Here's how the part is built. I have some questions about the finished solid (model axes, mm). A direction names the side the tool comes from. Coordinates: 2 decimals unless noted, no trailing zeros. Write each loop counter-clockwise with the first axis right and the second up, starting at its lowest first coordinate (ties: lowest second). Pieces come first, ordered by that corner, then holes. Notation, with made-up numbers: M 68.5,-35 L 102.5,-35 A30 ccw 102.5,-6 Z; hole C -23.5,29 d8. An arc over 180 degrees is marked long. Use one line per item in the form item = value. Start each with the question number.
1. On a 3-axis mill with a long thin cutter (end or side, diameter ignored), from which of +Z, -Z, +X, -X, +Y, -Y can I reach the whole of each face in a straight line? I mean faces 1 (the face through (-3.84, -3.97, -6.54)), 2 (the face through (-54, -1, -10)), 3 (the face through (-107.134, -8.541, -8.468)), 4 (the face through (2.51, 2.24, -8.47)), 5 (the face through (-53, -1, -13)). Say none if no direction works.
2. I want a section at B-B, the plane x = -19.5. List the corners of the cut face in (y, z) for me, plus the area to 3 significant figures.
3. Please list where these lines run through material, in increasing order: line 1 along Z through (x, y) = (-76.5, -0.5); line 2 along X through (y, z) = (-0.25, -1) (3 decimals); line 3 along Y through (x, z) = (-60, -11.5). Write a range as [from, to].
4. I'm going to push flat-ended pins straight in: pin 1 Ø1.1 at (x, z) = (-5.5, -6.5) entering from -Y; pin 2 Ø1.4 at (x, y) = (-109.5, -8) entering from -Z; pin 3 Ø8 at (y, z) = (-5.5, -9.5) entering from +X. Where does each tip first touch, or does it pass through?
5. Thinking about a two-plate mould opening in Y: for faces 6 (the face through (-108.25, -4, -9)), 7 (the face through (-109, -4, -10.75)), 8 (the face through (-55, -2, -11)), which applies, released by +Y, released by -Y, zero draft, split by the parting line, or undercut?
6. I want a section at C-C, the plane y = -3.5. List the corners of the cut face in (x, z) for me, plus the area to 3 significant figures.
7. I want a section at A-A, the plane z = -2.25. List the corners of the cut face in (x, y) for me (3 decimals).
Autodesk Inventor part; units mm, degrees
ref_plane "YZ Plane" through (0, 0, 0) normal (1, 0, 0) x (0, 1, 0)
ref_plane "XZ Plane" through (0, 0, 0) normal (0, 1, 0) x (-1, 0, 0)
ref_plane "XY Plane" through (0, 0, 0) normal (0, 0, 1) x (1, 0, 0)
sketch "Skizze1" plane through (0, 0, 0) normal (0, 1, 0) x (-1, 0, 0)
  line L0 (0, 0) -> (108, 0)
  line L1 (108, 0) -> (108, -15)
  line L2 (108, -15) -> (0, -15)
  line L3 (0, -15) -> (0, 0)
  dimension "d0" = 108
  dimension "d1" = 15
extrude "Extrusion1" add sketch "Skizze1" along normal blind 3
sketch "Skizze2" plane through (0, 0, 0) normal (0, -1, 0) x (1, 0, 0)
  line L0 (-108, 0) -> (0, 0)
  line L1 (-106.35, 0) -> (-1.65, 0)
  line L2 (-1.65, 0) -> (-1.65, 2)
  line L3 (-1.65, 2) -> (-106.35, 2)
  line L4 (-106.35, 2) -> (-106.35, 0)
  line L5 (-108, -15) -> (-108, 0)
  line L6 (0, -15) -> (-108, -15)
  line L7 (-54, -15) -> (-54, 78)
  point P0 (-54, 0)
  point P1 (-54, 2)
  dimension "d4" = 1.65
  dimension "d5" = 2
extrude "Extrusion2" add sketch "Skizze2" against normal blind 1.35 contours L4 L3 L7 L0 | L7 L3 L2 L0
sketch "Skizze3" plane through (0, 0, 0) normal (0, -1, 0) x (1, 0, 0)
  line L0 (0, -15) -> (-108, -15)
  line L1 (-106.65, -15) -> (-1.35, -15)
  line L2 (-1.35, -15) -> (-1.35, -13)
  line L3 (-1.35, -13) -> (-106.65, -13)
  line L4 (-106.65, -13) -> (-106.65, -15)
  line L5 (-54, -15) -> (-54, 54)
  line L6 (-108, -15) -> (-108, 0)
  point P0 (0, 0)
  dimension "d8" = 1.35
  dimension "d9" = 2
extrude "Extrusion3" cut sketch "Skizze3" against normal blind 1.65
ref_plane "Arbeitsebene1" through (0, 3, -10) normal (0, 0, -1) x (-1, 0, 0)
sketch "Skizze4" plane through (0, 0, 0) normal (0, -1, 0) x (1, 0, 0)
  line L0 (21.6, -10) -> (-129.6, -10)
  line L1 (-104.875, -10) -> (-3.125, -10)
  line L2 (-3.125, -10) -> (-3.125, -13)
  line L3 (-3.125, -13) -> (-104.875, -13)
  line L4 (-104.875, -13) -> (-104.875, -10)
  line L5 (-106.65, -13) -> (-1.35, -13)
  line L6 (-1.35, -13) -> (-1.35, -15)
  line L7 (0, -15) -> (-108, -15)
  line L8 (-54, -15) -> (-54, 34)
  point P0 (0, 0)
  point P1 (-3.125, -10)
  dimension "d36" = 101.75
extrude "Extrusion4" add sketch "Skizze4" along normal blind 2 contours L2 L3 L8 L0 | L8 L3 L4 L0
sketch "Skizze5" plane through (0, 0, 0) normal (0, -1, 0) x (1, 0, 0)
  line L0 (-3.125, -8.02) -> (-104.875, -8.02)
  line L1 (-104.875, -8.02) -> (-104.875, 2)
  line L2 (-104.875, 2) -> (-3.125, 2)
  line L3 (-3.125, 2) -> (-3.125, -8.02)
  line L4 (-3.125, -10) -> (-104.875, -10)
  line L5 (-104.875, -10) -> (-104.875, -13)
  line L6 (-3.125, -13) -> (-3.125, -10)
  line L7 (-1.65, 2) -> (-106.35, 2)
  point P0 (0, 0)
  dimension "d16" = 1.98
extrude "Extrusion5" add sketch "Skizze5" along normal up to surface (2 mm away)
sketch "Skizze6" plane through (-108, 0, -15) normal (-1, 0, 0) x (0, 0, 1)
  line L0 (15, 3) -> (0, 3)
  line L1 (0, 3) -> (15, 3)
  line L2 (15, 3) -> (15, 0)
  line L3 (15, 0) -> (0, 0)
  line L4 (0, 0) -> (0, 3)
extrude "Extrusion6" add sketch "Skizze6" along normal blind 1.5
sketch "Skizze9" plane through (0, 0, 0) normal (1, 0, 0) x (0, 0, -1)
  line L0 (0, 0) -> (15, 0)
  line L1 (15, 0) -> (15, 3)
  line L2 (0, 3) -> (15, 3)
  line L3 (0, 0) -> (0, 3)
extrude "Extrusion9" add sketch "Skizze9" along normal blind 1.5
sketch "Skizze7" plane through (-109.5, 0, -15) normal (-1, 0, 0) x (0, 0, 1)
  line L0 (15, 0) -> (0, 0)
  line L1 (4, 0) -> (9, 0) construction
  line L2 (9, 0) -> (9, -10) construction
  line L3 (9, -10) -> (4, -10) construction
  line L4 (4, -10) -> (4, 0) construction
  line L5 (0, 3) -> (0, 0)
  line L6 (4.25, 0) -> (8.75, 0)
  line L7 (8.75, 0) -> (8.75, -10.25)
  line L8 (8.75, -10.25) -> (4.25, -10.25)
  line L9 (4.25, -10.25) -> (4.25, 0)
  point P0 (9, 0)
  point P1 (8.75, 0)
  point P2 (4.25, 0)
  dimension "d22" = 4
  dimension "d23" = 5
  dimension "d24" = 10
  dimension "d37" = 0.25
  dimension "d38" = 0.25
  dimension "d39" = 0.25
extrude "Extrusion7" add sketch "Skizze7" against normal blind 1.25
extrude "Extrusion11" add sketch "Skizze7" along normal blind 1.25 from surface at -111
sketch "Skizze8" plane through (-109.5, -10, -6.25) normal (0, 0, 1) x (1, 0, 0)
  line L0 (0, 13) -> (111, 13)
  line L1 (55.5, 13) -> (55.5, -32)
  line L2 (0, -0.25) -> (0, 10)
  line L3 (0, -0.25) -> (1.25, -0.25)
  line L4 (1.25, 10) -> (1.25, -0.25)
  line L5 (0, 10) -> (1.25, 10)
  line L6 (0, -0.25) -> (0, 10)
  line L7 (1.25, 10) -> (1.25, -0.25)
  line L8 (111, -0.25) -> (111, 10)
  arc A0 (2.75, -0.25) -> (1.25, 2.8725) centre (-1.25, -0.25) ccw
  arc A1 (0, -0.25) -> (2.75, -0.25) centre (1.375, -0.25) ccw
  line L9 (0, -0.25) -> (1.25, -0.25)
  line L10 (1.25, 2.8725) -> (0, 2.8725)
  line L11 (0, -0.25) -> (0, 2.8725)
  line L12 (111, -0.25) -> (109.75, -0.25)
  arc A2 (109.75, 2.8725) -> (108.25, -0.25) centre (112.25, -0.25) ccw
  arc A3 (108.25, -0.25) -> (111, -0.25) centre (109.625, -0.25) ccw
  line L13 (111, -0.25) -> (109.75, -0.25)
  line L14 (109.75, 2.8725) -> (111, 2.8725)
  line L15 (111, -0.25) -> (111, 2.8725)
  point P0 (1.25, -4.25)
  point P1 (0, 2.8725)
  dimension "d76" = 4
  dimension "d77" = 1.5
extrude "Extrusion8" add sketch "Skizze8" against normal up to surface (4.5 mm away) contours L2 L10 L4 L3 | L3 L4 A0 A1 | A3 A2 L14 L8
sketch "Skizze11" plane through (0.25, 0, -6.25) normal (0, 0, 1) x (1, 0, 0)
  line L0 (1.25, 3) -> (-109.75, 3)
  line L1 (-54.25, 3) -> (-54.25, -19)
  line L2 (-109.75, 3) -> (1.25, 3)
  arc A0 (-1.5, -10.25) -> (1.25, -10.25) centre (-0.125, -10.25) ccw
  line L3 (1.25, -10.25) -> (3.25, 1.5)
  line L4 (3.25, 1.5) -> (1.25, 3)
  line L5 (1.25, 3) -> (1.25, 0)
  line L6 (1.25, 1.5) -> (5.25, 1.5) construction
  line L7 (1.25, -10.25) -> (1.25, 3) construction
  line L8 (1.25, -10.25) -> (1.25, 0) construction
  line L9 (-109.75, -10.25) -> (-111.75, 1.5)
  line L10 (-111.75, 1.5) -> (-109.75, 3)
  line L11 (-109.75, 3) -> (-109.75, 0)
  line L12 (-109.75, -10.25) -> (-109.75, 3) construction
  line L13 (-109.75, -10.25) -> (-109.75, 0) construction
  line L14 (1.25, -10.25) -> (1.25, 3)
  line L15 (-109.75, 0) -> (-109.75, 3)
  line L16 (-109.75, -10.25) -> (-109.75, 3)
  point P0 (-109.75, 1.5)
  point P1 (-109.75, 0)
  point P2 (1.25, 0)
  dimension "d78" = 2
extrude "Extrusion12" add sketch "Skizze11" against normal up to surface (4.5 mm away)
sketch "Skizze12" plane through (-1.35, 1.65, -13) normal (0, 0, -1) x (-1, 0, 0)
  line L0 (1.775, -1.65) -> (1.775, -3.65)
  line L1 (1.775, -3.65) -> (3.2309, -7.65)
  line L2 (3.2309, -7.65) -> (4.2309, -7.65)
  line L3 (4.2309, -7.65) -> (5.6868, -3.65)
  line L4 (103.525, -3.65) -> (1.775, -3.65)
  line L5 (-1.6, -15.9) -> (-3.35, -15.9)
  line L6 (-2.85, 1.35) -> (108.15, 1.35)
  line L7 (52.65, 1.35) -> (52.65, -27)
  line L8 (1.775, -3.65) -> (5.6868, -3.65)
  line L9 (103.525, -3.65) -> (102.0691, -7.65)
  line L10 (102.0691, -7.65) -> (101.0691, -7.65)
  line L11 (101.0691, -7.65) -> (99.6132, -3.65)
  line L12 (103.525, -3.65) -> (99.6132, -3.65)
  point P0 (-1.35, -1.65)
  dimension "d52" = 70
  dimension "d53" = 1
  dimension "d55" = 4
extrude "Extrusion13" add sketch "Skizze12" against normal up to surface (3 mm away)
extrude "Extrusion14" add sketch "Skizze12" against normal blind 3 from surface at -4.98
chamfer "Fasen2" distance 1 angle 45 4 edges at (-106.35, 0.675, 2) (-104.875, -1, 2) (-1.65, 0.675, 2) (-3.125, -1, 2)
ref_plane "Arbeitsebene2" through (1.5, 0, 0) normal (1, 0, 0) x (0, 0, -1)
sketch "Skizze13" plane through (1.5, 0, 0) normal (1, 0, 0) x (0, 0, -1)
  point P0 (0, 0)
sketch "Skizze14" plane through (1.5, 0, 0) normal (1, 0, 0) x (0, 0, -1)
  line L0 (-2, -2) -> (-1, -2)
  line L1 (-1, -2) -> (-2, -2)
  line L2 (5.02, -2) -> (-1, -2)
  line L3 (5.02, -2) -> (8.02, -2)
  line L4 (8.02, -2) -> (5.02, -2)
  line L5 (-1, -2) -> (5.02, -2)
  line L6 (10, -6) -> (10, -2)
  line L7 (10, -2) -> (10, -6)
  line L8 (10, 0) -> (10, -2)
  line L9 (10, 0) -> (10, -2)
  line L10 (10, -6) -> (10, -2)
  line L11 (10, -2) -> (10, -6)
  line L12 (0, 3) -> (6.25, 3)
  line L13 (6.25, 3) -> (0, 3)
  line L14 (10.75, 3) -> (6.25, 3)
  line L15 (15, 3) -> (10.75, 3)
  line L16 (10.75, 3) -> (15, 3)
  line L17 (6.25, 3) -> (10.75, 3)
  line L18 (10, -14.25) -> (1, -14.25)
  line L19 (1, -14.25) -> (1, 3)
  line L20 (1, 3) -> (10, 3)
  line L21 (10, 3) -> (10, -14.25)
  line L22 (10, 3) -> (12, 3)
  line L23 (12, 3) -> (12, -1)
  line L24 (12, -1) -> (10, -1)
  line L25 (10, -1) -> (10, 3)
  line L26 (1, 0.35) -> (-1.65, 3)
  line L27 (-1.65, 3) -> (1, 3)
  line L28 (-1, 1.35) -> (-2, 1.35)
  line L29 (-1, 1.35) -> (0, 1.35)
  line L30 (0, 1.35) -> (-1, 1.35)
  line L31 (-2, 1.35) -> (-1, 1.35)
  line L32 (0, 1.35) -> (1, 1.35) construction
  line L33 (6.25, -14.25) -> (10.75, -14.25)
  line L34 (6.25, -14.25) -> (10.75, -14.25)
  line L35 (6.25, -14.25) -> (10.75, -14.25)
  point P0 (0, 0)
  dimension "d64" = 9
  dimension "d65" = 2
  dimension "d66" = 4
  dimension "d67" = 45
  dimension "d69" = 1
equation "\"d0\" = Modul_Grundflächenlänge + 2 * Wandstärke"
equation "\"d1\" = Generische_Modulbreite"
equation "\"d2\" = Deckelstärke"
equation "\"d4\" = 0.55 * Basisstärke"
equation "\"d5\" = Modulüberlappung"
equation "\"d6\" = 0.45 * Deckelstärke"
equation "\"d8\" = 0.45 * Basisstärke"
equation "\"d9\" = Modulüberlappung"
equation "\"d10\" = 0.55 * Deckelstärke"
equation "\"d36\" = Modul_Grundflächenlänge - 0.5 * Stecktoleranz"
equation "\"d14\" = Deckel_Verstärkung"
equation "\"d16\" = 1.1 * Platinendicke"
equation "\"d20\" = Deckel_Klipperstärke"
equation "\"d31\" = Deckel_Klipperstärke"
equation "\"d22\" = Deckel_Klipperposition"
equation "\"d23\" = Deckel_Klippbreite"
equation "\"d24\" = Deckel_Klipplänge"
equation "\"d37\" = 0.5 * Stecktoleranz"
equation "\"d38\" = 0.5 * Stecktoleranz"
equation "\"d39\" = 0.5 * Stecktoleranz"
equation "\"d25\" = Deckel_Klipperstärke - 0.5 * Stecktoleranz"
equation "\"d40\" = Deckel_Klipperstärke - 0.5 * Stecktoleranz"
equation "\"d76\" = Deckelklipper_Radius"
equation "\"d77\" = Deckel_Klipptiefe"
equation "\"d55\" = Deckel_Einrastführungslänge"
equation "\"d64\" = Steckverbinder_Lochtiefe"
equation "\"d65\" = Steckverbinder_Absatzbreite"
equation "\"d66\" = Steckverbinder_Absatztiefe"
equation "\"Wandstärke\" = 3"
equation "\"Basisstärke\" = 3"
equation "\"Modulüberlappung\" = 2"
equation "\"Platinendicke\" = 1.8"
equation "\"Deckelstärke\" = 3"
equation "\"Seitenwand_Höhe\" = 39"
equation "\"Platinenposition\" = 5"
equation "\"d12\" = -Platinenposition"
equation "\"Deckel_Klippbreite\" = 5"
equation "\"Deckel_Klipplänge\" = 10"
equation "\"Deckel_Klipperposition\" = 4"
equation "\"Deckel_Klipperstärke\" = 1.5"
equation "\"Deckel_Klipptiefe\" = 1.5"
equation "\"Modul_Klipptiefe\" = 1.5"
equation "\"Modul_Klipperstärke\" = 1.5"
equation "\"Modul_Klipperposition\" = 7"
equation "\"Modul_Klipplänge\" = 8"
equation "\"Lüftungsraster\" = 2"
equation "\"Dings\" = 2"
equation "\"Modul_Grundflächenlänge\" = 102"
equation "\"Relais_Modulbreite\" = 28"
equation "\"Generische_Modulbreite\" = 15"
equation "\"Steckverbinderabsatztiefe\" = 4"
equation "\"Steckverbinder_Absatztiefe\" = 4"
equation "\"Steckverbinder_Absatzbreite\" = 2"
equation "\"Steckverbinder_Lochtiefe\" = 9"
equation "\"Steckverbinder_Fasenbreite\" = 1"
equation "\"Hauptmodul_Klipperabstand\" = 15"
equation "\"Stecktoleranz\" = 0.5"
equation "\"Rahmen_Durchbiegungsstopp\" = 5"
equation "\"Deckel_Einrastführungslänge\" = 4"
equation "\"Deckel_Verstärkung\" = 2"
equation "\"Deckelklipper_Radius\" = 4"
equation "\"Montage_Langloch\" = 5"
equation "\"Montage_Modulbreite\" = 15"
equation "\"Deckklipper_Kantenverrundung\" = 1"
equation "\"Montage_Bohrung\" = 4.5"
equation "\"Hauptmodul_Stufenposition\" = 53"
equation "\"Hauptmodulbreite\" = 28"
equation "\"Hauptmodul_Platinenhöhe_lang\" = 61"
equation "\"Hauptmodul_Platinenhöhe_kurz\" = 48"
equation "\"Generische_Platinenhöhe\" = 38"
equation "\"Modul_Klipperradius\" = 2"
equation "\"Modul_Klipper_Kantenverrundung\" = 1"
equation "\"Test_Schnittabstand\" = 5"
equation "\"Montage_Schwalbenschwanz_Winkel\" = 30deg"
equation "\"Montage_Schwalbenschwanz_Länge\" = 3"
equation "\"Hauptmodul_Deckel_Einschubtiefe\" = 2"
properties part number "Generischer Gehäuse Deckel"
Answer list:
q1.face_1 = +Z, -Z, -Y
q1.face_2 = -Y
q1.face_3 = +Z, -Z
q1.face_4 = +Z, -Z, +X, +Y
q1.face_5 = -Z, -Y
q2.outline = M -2,-13 L 1.65,-13 L 1.65,-15 L 3,-15 L 3,0 L 1.35,0 L 1.35,2 L -2,2 L -2,-8.02 L 0,-8.02 L 0,-10 L -2,-10 Z
q2.area = 70.4 mm²
q3.line_1 = [-13, -10], [-8.02, 2]
q3.line_2 = [-104.875, -3.125]
q3.line_3 = [-2, 3]
q4.pin_1 = -6
q4.pin_2 = -10.75
q4.pin_3 = 2.99
q5.face_6 = undercut
q5.face_7 = zero draft
q5.face_8 = released by -Y
q6.outline = M -110.65,-10.75 L -108.25,-10.75 L -108.25,-6.25 L -110.65,-6.25 Z; M -104.33,-13 L -101.51,-13 L -101.51,-10 L -104.33,-10 Z; M -104.33,-8.02 L -101.51,-8.02 L -101.51,-5.02 L -104.33,-5.02 Z; M -6.49,-13 L -3.67,-13 L -3.67,-10 L -6.49,-10 Z; M -6.49,-8.02 L -3.67,-8.02 L -3.67,-5.02 L -6.49,-5.02 Z; M 0.25,-10.75 L 2.65,-10.75 L 2.65,-6.25 L 0.25,-6.25 Z
q6.area = 55.4 mm²
q7.outline = M -109.5,0 L -104.875,0 L -104.875,-2 L -3.125,-2 L -3.125,0 L 1.5,0 L 1.5,3 L -109.5,3 Z
